from build123d import *

# Parameters (mm, degrees)
SKETCH006_R     = 115
PAD002_DEPTH    = 2
SKETCH007_R     = 83.5
POCKET001_DEPTH = 5
SKETCH008_R     = 2.1
POCKET002_DEPTH = 5
SKETCH009_R     = 4.5
SKETCH009_R_2   = 2.1
PAD008_DEPTH    = 3
POCKET013_DEPTH = 3.7


with BuildPart() as part:
    # Sketch006 → Pad002 (new body)
    with BuildSketch(Plane.XY):
        Circle(SKETCH006_R)
    extrude(amount=PAD002_DEPTH)

    # Sketch007 (on Face3 of Pad002) → Pocket001 (cut)
    with BuildSketch(Plane.XY.offset(2)):
        Circle(SKETCH007_R)
    extrude(amount=-POCKET001_DEPTH, mode=Mode.SUBTRACT)

    # Sketch008 (on Face3 of Pocket001) → Pocket002 (cut)
    with BuildSketch(Plane.XY.offset(2)):
        with Locations((15.447872, 97.534217)):
            Circle(SKETCH008_R)
        with Locations((58.043797, 79.890427)):
            Circle(SKETCH008_R)
        with Locations((79.890404, 58.043835)):
            Circle(SKETCH008_R)
        with Locations((97.534243, 15.447889)):
            Circle(SKETCH008_R)
        with Locations((15.447872, -97.534217)):
            Circle(SKETCH008_R)
        with Locations((58.043797, -79.890427)):
            Circle(SKETCH008_R)
        with Locations((79.890404, -58.043835)):
            Circle(SKETCH008_R)
        with Locations((97.534243, -15.447889)):
            Circle(SKETCH008_R)
        with Locations((-15.447872, 97.534217)):
            Circle(SKETCH008_R)
        with Locations((-58.043797, 79.890427)):
            Circle(SKETCH008_R)
        with Locations((-79.890404, 58.043835)):
            Circle(SKETCH008_R)
        with Locations((-97.534243, 15.447889)):
            Circle(SKETCH008_R)
        with Locations((-15.447872, -97.534217)):
            Circle(SKETCH008_R)
        with Locations((-58.043797, -79.890427)):
            Circle(SKETCH008_R)
        with Locations((-79.890404, -58.043835)):
            Circle(SKETCH008_R)
        with Locations((-97.534243, -15.447889)):
            Circle(SKETCH008_R)
    extrude(amount=-POCKET002_DEPTH, mode=Mode.SUBTRACT)

    # Sketch009 (on Face3 of Pocket002) → Pad008 (join)
    with BuildSketch(Plane.XY.offset(2)):
        with Locations((15.447874, 97.534228)):
            Circle(SKETCH009_R)
        with Locations((15.447874, 97.534228)):
            Circle(SKETCH009_R_2, mode=Mode.SUBTRACT)
        with Locations((58.043777, 79.890442)):
            Circle(SKETCH009_R)
        with Locations((58.043777, 79.89044)):
            Circle(SKETCH009_R_2, mode=Mode.SUBTRACT)
        with Locations((79.890404, 58.043831)):
            Circle(SKETCH009_R)
        with Locations((79.890401, 58.043831)):
            Circle(SKETCH009_R_2, mode=Mode.SUBTRACT)
        with Locations((97.534218, 15.447939)):
            Circle(SKETCH009_R)
        with Locations((97.534218, 15.447939)):
            Circle(SKETCH009_R_2, mode=Mode.SUBTRACT)
        with Locations((15.447874, -97.534228)):
            Circle(SKETCH009_R)
        with Locations((15.447874, -97.534228)):
            Circle(SKETCH009_R_2, mode=Mode.SUBTRACT)
        with Locations((58.043777, -79.890442)):
            Circle(SKETCH009_R)
        with Locations((58.043777, -79.89044)):
            Circle(SKETCH009_R_2, mode=Mode.SUBTRACT)
        with Locations((79.890404, -58.043831)):
            Circle(SKETCH009_R)
        with Locations((79.890401, -58.043831)):
            Circle(SKETCH009_R_2, mode=Mode.SUBTRACT)
        with Locations((97.534218, -15.447939)):
            Circle(SKETCH009_R)
        with Locations((97.534218, -15.447939)):
            Circle(SKETCH009_R_2, mode=Mode.SUBTRACT)
        with Locations((-15.447874, 97.534228)):
            Circle(SKETCH009_R)
        with Locations((-15.447874, 97.534228)):
            Circle(SKETCH009_R_2, mode=Mode.SUBTRACT)
        with Locations((-58.043777, 79.890442)):
            Circle(SKETCH009_R)
        with Locations((-58.043777, 79.89044)):
            Circle(SKETCH009_R_2, mode=Mode.SUBTRACT)
        with Locations((-79.890404, 58.043831)):
            Circle(SKETCH009_R)
        with Locations((-79.890401, 58.043831)):
            Circle(SKETCH009_R_2, mode=Mode.SUBTRACT)
        with Locations((-97.534218, 15.447939)):
            Circle(SKETCH009_R)
        with Locations((-97.534218, 15.447939)):
            Circle(SKETCH009_R_2, mode=Mode.SUBTRACT)
        with Locations((-15.447874, -97.534228)):
            Circle(SKETCH009_R)
        with Locations((-15.447874, -97.534228)):
            Circle(SKETCH009_R_2, mode=Mode.SUBTRACT)
        with Locations((-58.043777, -79.890442)):
            Circle(SKETCH009_R)
        with Locations((-58.043777, -79.89044)):
            Circle(SKETCH009_R_2, mode=Mode.SUBTRACT)
        with Locations((-79.890404, -58.043831)):
            Circle(SKETCH009_R)
        with Locations((-79.890401, -58.043831)):
            Circle(SKETCH009_R_2, mode=Mode.SUBTRACT)
        with Locations((-97.534218, -15.447939)):
            Circle(SKETCH009_R)
        with Locations((-97.534218, -15.447939)):
            Circle(SKETCH009_R_2, mode=Mode.SUBTRACT)
    extrude(amount=PAD008_DEPTH)

    # Sketch036 (on Face2 of Pad008) → Pocket013 (cut)
    with BuildSketch(Plane(origin=(0, 0, 0), x_dir=(1, 0, 0), z_dir=(0, 0, -1))):
        Polygon((14.800221, 93.567508), (18.721258, 95.072655), (19.378282, 99.220946), (16.114268, 101.864091), (12.193231, 100.358944), (11.536207, 96.210653), align=None)
        Polygon((55.599691, 76.542655), (59.776683, 76.103636), (62.24538, 79.501508), (60.537086, 83.338398), (56.360094, 83.777417), (53.891396, 80.379545), align=None)
        Polygon((76.462278, 55.553152), (80.29917, 53.84486), (83.69704, 56.31356), (83.258019, 60.490551), (79.421127, 62.198844), (76.023257, 59.730144), align=None)
        Polygon((93.227012, 14.730983), (95.870159, 11.466971), (100.018449, 12.123997), (101.523593, 16.045036), (98.880446, 19.309048), (94.732156, 18.652022), align=None)
        Polygon((-14.800222, 93.567508), (-18.721259, 95.072655), (-19.378283, 99.220946), (-16.114269, 101.864091), (-12.193232, 100.358944), (-11.536208, 96.210653), align=None)
        Polygon((-55.599691, 76.542655), (-59.776683, 76.103636), (-62.245381, 79.501508), (-60.537086, 83.338398), (-56.360094, 83.777417), (-53.891397, 80.379545), align=None)
        Polygon((-76.462278, 55.553152), (-80.29917, 53.84486), (-83.69704, 56.31356), (-83.258019, 60.490551), (-79.421127, 62.198844), (-76.023257, 59.730144), align=None)
        Polygon((-93.227012, 14.730983), (-95.870158, 11.466971), (-100.018449, 12.123998), (-101.523593, 16.045036), (-98.880446, 19.309048), (-94.732156, 18.652022), align=None)
        Polygon((14.800222, -93.567508), (18.721259, -95.072655), (19.378283, -99.220946), (16.114269, -101.864091), (12.193232, -100.358944), (11.536208, -96.210653), align=None)
        Polygon((55.599691, -76.542655), (59.776683, -76.103636), (62.245381, -79.501508), (60.537086, -83.338398), (56.360094, -83.777417), (53.891397, -80.379545), align=None)
        Polygon((76.462278, -55.553152), (80.29917, -53.84486), (83.69704, -56.31356), (83.258019, -60.490551), (79.421127, -62.198844), (76.023257, -59.730144), align=None)
        Polygon((93.227012, -14.730983), (95.870158, -11.466971), (100.018449, -12.123998), (101.523593, -16.045036), (98.880446, -19.309048), (94.732156, -18.652022), align=None)
        Polygon((-14.800222, -93.567508), (-18.721259, -95.072655), (-19.378283, -99.220946), (-16.114269, -101.864091), (-12.193232, -100.358944), (-11.536208, -96.210653), align=None)
        Polygon((-55.599691, -76.542655), (-59.776683, -76.103636), (-62.245381, -79.501508), (-60.537086, -83.338398), (-56.360094, -83.777417), (-53.891397, -80.379545), align=None)
        Polygon((-76.462278, -55.553152), (-80.29917, -53.84486), (-83.69704, -56.31356), (-83.258019, -60.490551), (-79.421127, -62.198844), (-76.023257, -59.730144), align=None)
        Polygon((-93.227012, -14.730983), (-95.870158, -11.466971), (-100.018449, -12.123998), (-101.523593, -16.045036), (-98.880446, -19.309048), (-94.732156, -18.652022), align=None)
    extrude(amount=-POCKET013_DEPTH, mode=Mode.SUBTRACT)


with BuildPart() as part_1:
    # Body003 placement: moved
    add(part.part.moved(Location((0, 0, 8.7))))


solid = part_1.part
The model under review builds one solid part; all positions refer to its coordinate system, in mm. A direction names the side the tool comes from. Give positions to 0.01 mm unless a question says otherwise; leave off trailing zeros. Loops run counter-clockwise (first coordinate to the right, second up) from the corner with the lowest first, then second, coordinate; pieces in that order, holes last. Notation, with made-up numbers: (49, -4) -> (84, -4) arc R37 ccw to (84, 32) -> close; hole circle Ø11 at (49, -8.5). An arc over 180 degrees is marked (long way). Write each question's results on one line, items separated by ' | '.
1) Draft analysis for pull direction X (two halves, no side actions). For faces 1 (the face through (95.6, 17.1, 12.4)), 2 (the face through (-81, 56, 13.7)), state which applies: pulls with the +X half, pulls with the -X half, needs draft (parallel to the pull), parting line crosses it, or undercut.
Conclusion:
face 1: undercut | face 2: needs draft
2) Take a section at A-A, the plane y = 0. Give the boundary of the cut face in (x, z).
Conclusion:
outline: (-115, 8.7) -> (-83.5, 8.7) -> (-83.5, 10.7) -> (-115, 10.7) -> close; (83.5, 8.7) -> (115, 8.7) -> (115, 10.7) -> (83.5, 10.7) -> close
3) For line 1 along Y through (x, z) = (-62, 12.45); line 2 along X through (y, z) = (-15, 11.1); line 3 along X through (y, z) = (-16.5, 10.45), list the stretches that pass through material, from the lowest coordinate up. Write a range as from..to.
Conclusion:
line 1: y = -82.03..-77.75, 77.75..82.03 | line 2: x = -102.01..-101.12, -93.33..-93.06, 93.06..93.33, 101.12..102.01 | line 3: x = -113.81..-101.16, -93.91..-81.85, 81.85..93.91, 101.16..113.81
4) Insertion check: pin 1 Ø12 at (x, y) = (51, -64) entering from +Z; pin 2 Ø1.5 at (y, z) = (27, 9.5) entering from -X; pin 3 Ø2.5 at (x, y) = (-79.5, -56) entering from -Z. Each pin has a flat end and moves straight along its axis. Give the tip position at first contact, or say it passes through.
Conclusion:
pin 1: stops at z = 10.7 | pin 2: stops at x = -111.96 | pin 3: stops at z = 12.4
5) Take a section at C-C, the plane x = -89. Give the boundary of the cut face in (y, z).
Conclusion:
outline: (-72.83, 8.7) -> (72.83, 8.7) -> (72.83, 10.7) -> (-72.83, 10.7) -> close
6) Tool access review of faces 3 (the face through (-95.6, 17.1, 12.4)), 4 (the face through (13, -98, 13.7)), 5 (the face through (-13.371, -101.527, 12.179)): name each direction out of +Z, -Z, +X, -X, +Y, -Y from which nothing blocks a thin tool from reaching the whole face with its end or side.
Conclusion:
face 3: -Z | face 4: +Z, +X, -X, +Y, -Y | face 5: +Z
